Build history of the part. All positions in model axes, mm. A direction names the side the tool comes from. Round coordinates to 2 decimals unless told otherwise and drop trailing zeros. Loops run counter-clockwise (first coordinate to the right, second up) from the corner with the lowest first, then second, coordinate; pieces in that order, holes last. Notation, with made-up numbers: (60.5, 37) - (73.5, 37) arc R21 cw to (73.5, 49) - close; hole circle Ø4 at (-37.5, 76.5). An arc over 180 degrees is marked (long way). Answer as CSV lines item,"result". Start each with the question number.
```python
from build123d import *

# Parameters (mm, degrees)
SK_P01_STANDOFF_R        = 2.5
P01_STANDOFF_DEPTH       = 6
SK_P02_STANDOFF_R        = 2.5
P02_STANDOFF_DEPTH       = 6
SK_P03_STANDOFF_R        = 2.5
P03_STANDOFF_DEPTH       = 6
SK_P04_STANDOFF_R        = 2.5
P04_STANDOFF_DEPTH       = 6
P05_BOARD_START          = 6
SK_P05_BOARD_W           = 85
SK_P05_BOARD_H           = 56
P05_BOARD_DEPTH          = 1.6
P06_ACTIVECOOLER_START   = 7.6
SK_P06_ACTIVECOOLER_W    = 40
SK_P06_ACTIVECOOLER_H    = 40
P06_ACTIVECOOLER_DEPTH   = 10
P07_USBANDETHERNET_START = 7.6
SK_P07_USBANDETHERNET_W  = 17.5
SK_P07_USBANDETHERNET_H  = 53
P07_USBANDETHERNET_DEPTH = 16
P08_USBCPOWER_START      = 7.6
SK_P08_USBCPOWER_W       = 6.5
SK_P08_USBCPOWER_H       = 7
P08_USBCPOWER_DEPTH      = 3.2
P09_MICROHDMI0_START     = 7.6
SK_P09_MICROHDMI0_W      = 6.4
SK_P09_MICROHDMI0_H      = 7
P09_MICROHDMI0_DEPTH     = 3
P10_MICROHDMI1_START     = 7.6
SK_P10_MICROHDMI1_W      = 6.4
SK_P10_MICROHDMI1_H      = 7
P10_MICROHDMI1_DEPTH     = 3


with BuildPart() as part:
    # SK_P01_Standoff → P01_Standoff (new body)
    with BuildSketch(Plane(origin=(0, 0, 0), x_dir=(1, 0, 0), z_dir=(0, 1, 0))):
        with Locations(Location((-19, 24.5, 0), (0, 0, 270))):
            Circle(SK_P01_STANDOFF_R)
    extrude(amount=P01_STANDOFF_DEPTH)



with BuildPart() as body_2:
    # SK_P02_Standoff → P02_Standoff (new body)
    with BuildSketch(Plane(origin=(0, 0, 0), x_dir=(1, 0, 0), z_dir=(0, 1, 0))):
        with Locations(Location((-19, -24.5, 0), (0, 0, 270))):
            Circle(SK_P02_STANDOFF_R)
    extrude(amount=P02_STANDOFF_DEPTH)


with BuildPart() as body_3:
    # SK_P03_Standoff → P03_Standoff (new body)
    with BuildSketch(Plane(origin=(0, 0, 0), x_dir=(1, 0, 0), z_dir=(0, 1, 0))):
        with Locations(Location((39, 24.5, 0), (0, 0, 270))):
            Circle(SK_P03_STANDOFF_R)
    extrude(amount=P03_STANDOFF_DEPTH)


with BuildPart() as body_4:
    # SK_P04_Standoff → P04_Standoff (new body)
    with BuildSketch(Plane(origin=(0, 0, 0), x_dir=(1, 0, 0), z_dir=(0, 1, 0))):
        with Locations(Location((39, -24.5, 0), (0, 0, 270))):
            Circle(SK_P04_STANDOFF_R)
    extrude(amount=P04_STANDOFF_DEPTH)


with BuildPart() as part_1:
    add(part.part)

    add(body_2.part)  # P05_Board merges body 2

    add(body_3.part)  # P05_Board merges body 3

    add(body_4.part)  # P05_Board merges body 4
    # SK_P05_Board → P05_Board (add)
    with BuildSketch(Plane(origin=(0, 0, 0), x_dir=(1, 0, 0), z_dir=(0, 1, 0)).offset(P05_BOARD_START)):
        Rectangle(SK_P05_BOARD_W, SK_P05_BOARD_H)
    extrude(amount=P05_BOARD_DEPTH)

    # SK_P06_Activecooler → P06_Activecooler (add)
    with BuildSketch(Plane(origin=(0, 0, 0), x_dir=(1, 0, 0), z_dir=(0, 1, 0)).offset(P06_ACTIVECOOLER_START)):
        with Locations((5, 0)):
            Rectangle(SK_P06_ACTIVECOOLER_W, SK_P06_ACTIVECOOLER_H)
    extrude(amount=P06_ACTIVECOOLER_DEPTH)

    # SK_P07_USBandEthernet → P07_USBandEthernet (add)
    with BuildSketch(Plane(origin=(0, 0, 0), x_dir=(1, 0, 0), z_dir=(0, 1, 0)).offset(P07_USBANDETHERNET_START)):
        with Locations((-33.75, 0)):
            Rectangle(SK_P07_USBANDETHERNET_W, SK_P07_USBANDETHERNET_H)
    extrude(amount=P07_USBANDETHERNET_DEPTH)

    # SK_P08_USBCpower → P08_USBCpower (add)
    with BuildSketch(Plane(origin=(0, 0, 0), x_dir=(1, 0, 0), z_dir=(0, 1, 0)).offset(P08_USBCPOWER_START)):
        with Locations((31.25, 24.5)):
            Rectangle(SK_P08_USBCPOWER_W, SK_P08_USBCPOWER_H)
    extrude(amount=P08_USBCPOWER_DEPTH)

    # SK_P09_microHDMI0 → P09_microHDMI0 (add)
    with BuildSketch(Plane(origin=(0, 0, 0), x_dir=(1, 0, 0), z_dir=(0, 1, 0)).offset(P09_MICROHDMI0_START)):
        with Locations((16.7, 24.5)):
            Rectangle(SK_P09_MICROHDMI0_W, SK_P09_MICROHDMI0_H)
    extrude(amount=P09_MICROHDMI0_DEPTH)

    # SK_P10_microHDMI1 → P10_microHDMI1 (add)
    with BuildSketch(Plane(origin=(0, 0, 0), x_dir=(1, 0, 0), z_dir=(0, 1, 0)).offset(P10_MICROHDMI1_START)):
        with Locations((3.3, 24.5)):
            Rectangle(SK_P10_MICROHDMI1_W, SK_P10_MICROHDMI1_H)
    extrude(amount=P10_MICROHDMI1_DEPTH)


solid = part_1.part
```
Q1. Tool access for faces 1 (the flat face through (28, 9, -24)), 2 (the flat face through (5, 17.6, 0)), 3 (the flat face through (-34, 15, 26.5)), 4 (the flat face through (3, 10.6, -25)): list every direction of +Z, -Z, +X, -X, +Y, -Y with a clear straight run to the whole face (end or side of a thin tool).
Q2. Band-saw the part on C-C, the plane x = 39. List the corners of the cut face in (y, z), then the cut area to 3 significant figures.
Q3. Band-saw the part on D-D, the plane y = 2. List the corners of the cut face in (x, z), then the cut area to 3 significant figures.
Q4. Pin check, flat tips, straight feed: pin 1 Ø4 at (x, z) = (-8, 16) entering from -Y; pin 2 Ø1.9 at (x, z) = (3.5, -24.5) entering from +Y; pin 3 Ø5 at (x, y) = (2, 18.5) entering from +Z. Stop position of each tip, or through.
Q5. Band-saw the part on A-A, the plane y = 16.5. List the corners of the cut face in (x, z).
Q6. Wall check: probe 1 along X at (y, z) = (10, -22); probe 2 along X at (y, z) = (17.5, 11.5); probe 3 along Y at (x, z) = (24, 7). Give the ranges that are in metal, low to high. Write a range as [from, to].
Q7. Band-saw the part on B-B, the plane z = 24.5. List the corners of the cut face in (x, y), then the cut area to 3 significant figures.
Q8. Two-plate mould, pull along Z, no slides. Class faces 5 (the flat face through (3, 9, -21)), 6 (the flat face through (5, 13, 20)), 7 (the flat face through (13.5, 9, -24)): released by +Z, released by -Z, zero draft, split by the parting line, or undercut.
Reported:
1,face 1,"+Z, -Z, +Y"
1,face 2,"+Z, -Z, +X, +Y"
1,face 3,"+Z, +X, -X, +Y"
1,face 4,"-Z, +Y"
2,outline,"(0, -27) - (6, -27) - (6, -28) - (7.6, -28) - (7.6, 28) - (6, 28) - (6, 27) - (0, 27) - (0, 22) - (6, 22) - (6, -22) - (0, -22) - close"
2,area,"150 mm2"
3,outline,"circle Ø5 at (-19, -24.5); circle Ø5 at (-19, 24.5); circle Ø5 at (39, -24.5); circle Ø5 at (39, 24.5)"
3,area,"78.5 mm2"
4,pin 1,"stops at y = 6"
4,pin 2,"stops at y = 10.6"
4,pin 3,"stops at z = 20"
5,outline,"(-42.5, -26.5) - (-25, -26.5) - (-25, 26.5) - (-42.5, 26.5) - close; (-15, -20) - (25, -20) - (25, 20) - (-15, 20) - close"
6,probe 1,"x = [-42.5, -25], [0.1, 6.5], [13.5, 19.9], [28, 34.5]"
6,probe 2,"x = [-42.5, -25], [-15, 25]"
6,probe 3,"y = [6, 17.6]"
7,outline,"(-42.5, 6) - (-21.5, 6) - (-21.5, 0) - (-16.5, 0) - (-16.5, 6) - (36.5, 6) - (36.5, 0) - (41.5, 0) - (41.5, 6) - (42.5, 6) - (42.5, 7.6) - (-25, 7.6) - (-25, 23.6) - (-42.5, 23.6) - close"
7,area,"476 mm2"
8,face 5,"undercut"
8,face 6,"released by +Z"
8,face 7,"zero draft"
